The listing builds one solid part. Answer for the finished solid, in the listing's coordinates (mm). A direction names the side the tool comes from. Coordinates: 2 decimals unless noted, no trailing zeros. Write each loop counter-clockwise with the first axis right and the second up, starting at its lowest first coordinate (ties: lowest second). Pieces come first, ordered by that corner, then holes.
(1) Given P1, Ø5, axis at x = 18.5, z = 22, coming from the -Y side; P2, Ø3, axis at x = 16, z = 21.5, coming from the -Y side; P3, Ø2, axis at x = 11, z = 12, coming from the +Y side; P4, Ø6, axis at x = 0, y = 0, coming from the -Z side, each flat-ended and moving along its own axis, determine where each tip first touches the part or whether it passes through.
(2) The part is cut by section B-B on z = 18. Determine the outline of the cut face in (x, y), plus the area to 3 significant figures.
(3) The part is cut by section D-D on x = -27. Determine the outline of the cut face in (y, z).
(4) Which of the six approach directions +Z, -Z, +X, -X, +Y, -Y give full straight-line access (tool end or side, diameter ignored) to faces 1 (the flat face through (3.94, -26.29, 15.32)), 2 (the flat face through (11, -16, 3)), 3 (the flat face through (7, 0, 0)), 4 (the flat face through (-24.59, 10.49, 15.32)), 5 (the flat face through (24.59, -10.49, 15.32))?
(5) The part is cut by section A-A on y = 0. Determine the outline of the cut face in (x, z).
(6) For a pull along Z with two mould halves and no side action, classify faces 6 (the flat face through (-3.94, 26.29, 15.32)), 7 (the flat face through (0, 2.15, 14)), 8 (the flat face through (7, 0, 31)) as +Z half, -Z half, draft (parallel to the pull), parting line (faces both ways), or undercut.
(7) Straight lines are drawn through the part: line 1 (X direction, y = 0, z = 8.5); line 2 (Z direction, x = 26, y = -14); line 3 (X direction, y = -9, z = 15.5). For each, find the intervals that lie inside material, in ascending order.
(8) The part is cut by section C-C on y = -23. Determine the outline of the cut face in (x, z), plus the area to 3 significant figures.
from build123d import *

# Parameters (mm, degrees)
SKETCH2_R           = 32.5
BOSS_EXTRUDE1_DEPTH = 3
BOSS_EXTRUDE2_DEPTH = 25
SKETCH4_R           = 32.5
BOSS_EXTRUDE3_DEPTH = 3
CUT_EXTRUDE1_DEPTH  = 56.439155838
SKETCH7_R           = 2.65
CUT_EXTRUDE2_DEPTH  = 3


with BuildPart() as part:
    # Sketch2 → Boss-Extrude1 (new body)
    with BuildSketch(Plane.XY):
        Circle(SKETCH2_R)
    extrude(amount=BOSS_EXTRUDE1_DEPTH)

    # Sketch3 → Boss-Extrude2 (add)
    with BuildSketch(Plane.XY.offset(3)):
        with BuildLine():
            Line((0, 7.5), (0, 21.210393848))
            Line((0, 21.210393848), (-7.984489127, 31.503935205))
            ThreePointArc((-7.984489127, 31.503935205), (-4.023189397, 32.250022435), (0, 32.5))
            ThreePointArc((0, 32.5), (25.680037902, 19.919479244), (31.478952737, -8.082421333))
            ThreePointArc((31.478952737, -8.082421333), (30.23630216, -11.917047944), (28.528519449, -15.56835181))
            Line((28.528519449, -15.56835181), (20.544030322, -5.274810453))
            Line((20.544030322, -5.274810453), (7.264373708, -1.865174154))
            ThreePointArc((7.264373708, -1.865174154), (4.596802902, -5.926162593), (0, -7.5))
            Line((0, -7.5), (0, -21.210393848))
            Line((0, -21.210393848), (7.984489127, -31.503935205))
            ThreePointArc((7.984489127, -31.503935205), (4.023189397, -32.250022435), (0, -32.5))
            ThreePointArc((0, -32.5), (-25.680037902, -19.919479244), (-31.478952737, 8.082421333))
            ThreePointArc((-31.478952737, 8.082421333), (-30.23630216, 11.917047944), (-28.528519449, 15.56835181))
            Line((-28.528519449, 15.56835181), (-20.544030322, 5.274810453))
            Line((-20.544030322, 5.274810453), (-7.264373708, 1.865174154))
            ThreePointArc((-7.264373708, 1.865174154), (-4.596802902, 5.926162593), (0, 7.5))
        make_face()
    extrude(amount=BOSS_EXTRUDE2_DEPTH)

    # Sketch4 → Boss-Extrude3 (add)
    with BuildSketch(Plane.XY.offset(28)):
        Circle(SKETCH4_R)
    extrude(amount=BOSS_EXTRUDE3_DEPTH)

    # Sketch5 → Cut-Extrude1 (cut, through all)
    with BuildSketch(Plane.XY.offset(31)):
        with BuildLine():
            Line((-1.549193338, 2.15), (1.549193338, 2.15))
            ThreePointArc((1.549193338, 2.15), (0, -2.65), (-1.549193338, 2.15))
        make_face()
    extrude(amount=-CUT_EXTRUDE1_DEPTH, mode=Mode.SUBTRACT)

    # Sketch7 → Cut-Extrude2 (cut)
    with BuildSketch(Plane.XY.offset(31)):
        Circle(SKETCH7_R)
    extrude(amount=-CUT_EXTRUDE2_DEPTH, mode=Mode.SUBTRACT)


solid = part.part
Model answer:
1. P1: stops at y = -5.86
1. P2: stops at y = -4.49
1. P3: stops at y = 30.92
1. P4: stops at z = 0
2. outline: (-28.53, 15.57) arc R32.5 ccw to (7.98, -31.5) - (0, -21.21) - (0, -7.5) arc R7.5 ccw to (7.26, -1.87) - (20.54, -5.27) - (28.53, -15.57) arc R32.5 ccw to (-7.98, 31.5) - (0, 21.21) - (0, 7.5) arc R7.5 ccw to (-7.26, 1.87) - (-20.54, 5.27) - close; hole (-1.55, 2.15) arc R2.65 ccw (long way) to (1.55, 2.15) - close
2. area: 2,160 mm2
3. outline: (-18.09, 0) - (18.09, 0) - (18.09, 3) - (13.6, 3) - (13.6, 28) - (18.09, 28) - (18.09, 31) - (-18.09, 31) - close
4. face 1: +X
4. face 2: none
4. face 3: -Z, +X, -X, +Y, -Y
4. face 4: +Y
4. face 5: -Y
5. outline: (-32.5, 0) - (-2.65, 0) - (-2.65, 31) - (-32.5, 31) - close; (2.65, 0) - (32.5, 0) - (32.5, 31) - (2.65, 31) - close
6. face 6: undercut
6. face 7: draft
6. face 8: +Z half
7. line 1: x = -32.5 to -2.65, 2.65 to 32.5
7. line 2: z = 0 to 3, 28 to 31
7. line 3: x = -31.23 to 0, 23.43 to 31.23
8. outline: (-22.96, 0) - (22.96, 0) - (22.96, 3) - (1.39, 3) - (1.39, 28) - (22.96, 28) - (22.96, 31) - (-22.96, 31) - close
8. area: 884 mm2
